```python
from build123d import *

# Parameters (mm, degrees)
F1_DEPTH = 9.525
F2_R     = 4.7625
F2_R_2   = 2.286
F3_DEPTH = 25.4
F4_SIZE  = 5.08


with BuildPart() as f1:
    # F0 (on Top) → F1 (new body)
    with BuildSketch(Plane.XY):
        Polygon((0, 12.7), (0, 0), (44.45, 0), (44.45, 12.7), (31.75, 12.7), (31.75, 44.45), (12.7, 44.45), (12.7, 12.7), align=None)
    extrude(amount=F1_DEPTH)

    # F2 (on face) → F3 (cut)
    with BuildSketch(Plane.XY.offset(9.525)):
        with Locations((22.225, 31.75)):
            Circle(F2_R)
        with Locations((6.35, 6.35)):
            Circle(F2_R_2)
        with Locations((38.1, 6.35)):
            Circle(F2_R_2)
    extrude(amount=-F3_DEPTH, mode=Mode.SUBTRACT)

    # F4
    f4_edges = [f1.edges().sort_by_distance(p)[0] for p in [
        (12.7, 44.45, 4.7625),
        (31.75, 44.45, 4.7625),
    ]]
    chamfer(f4_edges, length=F4_SIZE)


solid = f1.part
```
Verification items for the finished model (mm, model axes). A direction names the side the tool comes from. Coordinates: 2 decimals unless noted, no trailing zeros. Order: outer loops, then holes, each group sorted by start corner. A loop starts at its lowest first (then second) coordinate and runs counter-clockwise, first axis right, second up. Notation, with made-up numbers: (3, -15) -> (44, -15) arc R13 cw to (44, 2) -> close; hole circle Ø6 at (87.25, -38). An arc over 180 degrees is marked (long way). Put each result on its own line as item: value. Start each with the question number.
1) Material ranges on L1, parallel to Y at x = 6.35, z = 6.5; L2, parallel to Y at x = 4, z = 3.75; L3, parallel to X at y = 16.5, z = 5.75, recorded low to high.
2) Release check for a two-part mould opening along Y. For faces 1 (the flat face through (29.25, 41.87, 4.7)), 2 (the cylindrical face through (7.579, 8.278, 4.829)), 3 (the flat face through (0, 6, 5)), 4 (the cylindrical face through (18.715, 34.969, 4.829)) record: pulls with the +Y half, pulls with the -Y half, needs draft (parallel to the pull), parting line crosses it, or undercut.
3) Cross-section at C-C (z = 5.5). State how many separate pieces and enclosed holes the cut face has, plus the area to 3 significant figures.
4) Cross-section at B-B (x = 38.1). Enter the section's corners in (y, z) (3 decimals), plus the area to 3 significant figures.
5) Cross-section at A-A (y = 6.35). Enter the section's corners in (x, z) (3 decimals), plus the area to 3 significant figures.
6) Go/stop test with flat-tipped pins: pin 1 (2.5 mm diameter, centred on x = 6.35, y = 6.35, fed in from +Z); pin 2 (5 mm diameter, centred on y = 20.5, z = 7, fed in from -X); pin 3 (4 mm diameter, centred on x = 36, z = 2, fed in from +Y). Record where each tip stops, or that it passes through.
7) Tool access check on faces 5 (the flat face through (12.7, 26, 5)), 6 (the flat face through (31.75, 26, 5)), 7 (the flat face through (22, 0, 5)). Record the directions out of +Z, -Z, +X, -X, +Y, -Y that give a thin tool (end or side, any length) a straight path to the whole face; none if there is none.
Geometry check:
1. L1: y = 0 to 4.06, 8.64 to 12.7
1. L2: y = 0 to 12.7
1. L3: x = 12.7 to 31.75
2. face 1: pulls with the +Y half
2. face 2: undercut
2. face 3: needs draft
2. face 4: undercut
3. separate pieces: 1
3. enclosed holes: 3
3. area: 1,040 mm^2
4. outline: (0, 0) -> (4.064, 0) -> (4.064, 9.525) -> (0, 9.525) -> close; (8.636, 0) -> (12.7, 0) -> (12.7, 9.525) -> (8.636, 9.525) -> close
4. area: 77.4 mm^2
5. outline: (0, 0) -> (4.064, 0) -> (4.064, 9.525) -> (0, 9.525) -> close; (8.636, 0) -> (35.814, 0) -> (35.814, 9.525) -> (8.636, 9.525) -> close; (40.386, 0) -> (44.45, 0) -> (44.45, 9.525) -> (40.386, 9.525) -> close
5. area: 336 mm^2
6. pin 1: passes through
6. pin 2: stops at x = 12.7
6. pin 3: stops at y = 12.7
7. face 5: +Z, -Z, -X, +Y
7. face 6: +Z, -Z, +X, +Y
7. face 7: +Z, -Z, +X, -X, -Y
